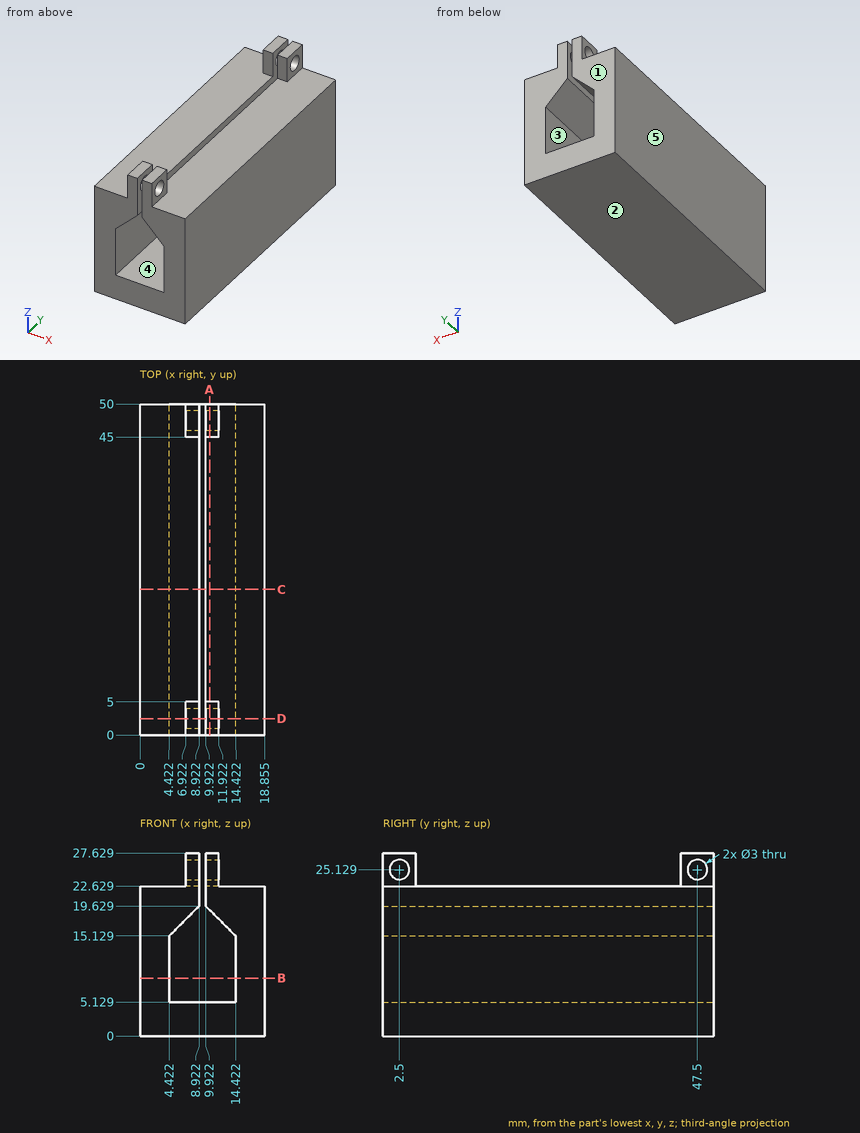
Part print with two shaded views. Sizes in mm from the minimum x, y, z corner. A direction names the side the tool comes from. Coordinates: 2 decimals unless noted, no trailing zeros. Loops run counter-clockwise (first coordinate to the right, second up) from the corner with the lowest first, then second, coordinate; pieces in that order, holes last. Notation, with made-up numbers: M -7,-13.75 L -2,-13.75 A15 cw -2,-1.75 Z; hole C 75,-27 d11. An arc over 180 degrees is marked long. Use CSV: the item, a comma, the result in double quotes. Start each with the question number.
1. Band-saw the part on C-C, the plane y = 22. List the corners of the cut face in (x, z) (1 decimal).
2. Flat gauge pins, fed straight in: pin 1 (1.5 mm diameter, centred on x = 12.5, y = 7, fed in from -Z); pin 2 (7 mm diameter, centred on x = 2.5, y = 21, fed in from +Z); pin 3 (1.5 mm diameter, centred on y = 48.5, z = 24.5, fed in from -X); pin 4 (5.5 mm diameter, centred on y = 2.5, z = 26, fed in from +X). Where does each tip first touch, or does it go through?
3. Band-saw the part on A-A, the plane x = 10.5. List the corners of the cut face in (y, z), then the cut area to 3 significant figures.
4. Band-saw the part on D-D, the plane y = 2.5. List the corners of the cut face in (x, z) (1 decimal).
5. Tool access for the marked faces 4 and 5: list every direction of +Z, -Z, +X, -X, +Y, -Y with a clear straight run to the whole face (end or side of a thin tool).
6. Two-plate mould, pull along Z, no slides. Class the marked faces 1, 2 and 3: pulls with the +Z half, pulls with the -Z half, needs draft (parallel to the pull), parting line crosses it, or undercut.
7. Probe probe 1 along X at (y, z) = (14, 6.5) (1 decimal); probe 2 along Y at (x, z) = (10, 25.75) (1 decimal); probe 3 along Z at (x, y) = (11.4, 47.5). List the from-to ranges inside material, lowest first. Write a range as [from, to].
8. Band-saw the part on B-B, the plane z = 8.75. List the corners of the cut face in (x, y) (1 decimal), then the cut area to 3 significant figures.
Entries:
1,outline,"M 0,0 L 18.9,0 L 18.9,22.6 L 9.9,22.6 L 9.9,19.6 L 14.4,15.1 L 14.4,5.1 L 4.4,5.1 L 4.4,15.1 L 8.9,19.6 L 8.9,22.6 L 0,22.6 Z"
2,pin 1,"stops at z = 0"
2,pin 2,"stops at z = 22.63"
2,pin 3,"stops at x = 6.92"
2,pin 4,"stops at x = 11.92"
3,outline,"M 0,0 L 50,0 L 50,5.13 L 0,5.13 Z; M 0,19.05 L 50,19.05 L 50,27.63 L 45,27.63 L 45,22.63 L 5,22.63 L 5,27.63 L 0,27.63 Z; hole C 2.5,25.13 d3; hole C 47.5,25.13 d3"
3,area,"471 mm2"
4,outline,"M 0,0 L 18.9,0 L 18.9,22.6 L 11.9,22.6 L 11.9,23.6 L 9.9,23.6 L 9.9,19.6 L 14.4,15.1 L 14.4,5.1 L 4.4,5.1 L 4.4,15.1 L 8.9,19.6 L 8.9,23.6 L 6.9,23.6 L 6.9,22.6 L 0,22.6 Z; M 6.9,26.6 L 8.9,26.6 L 8.9,27.6 L 6.9,27.6 Z; M 9.9,26.6 L 11.9,26.6 L 11.9,27.6 L 9.9,27.6 Z"
5,face 4,"+Y, -Y"
5,face 5,"+Z, -Z, -X, +Y, -Y"
6,face 1,"needs draft"
6,face 2,"pulls with the -Z half"
6,face 3,"undercut"
7,probe 1,"x = [0, 4.4], [14.4, 18.9]"
7,probe 2,"y = [0, 1.1], [3.9, 5], [45, 46.1], [48.9, 50]"
7,probe 3,"z = [0, 5.13], [18.15, 23.63], [26.63, 27.63]"
8,outline,"M 0,0 L 4.4,0 L 4.4,50 L 0,50 Z; M 14.4,0 L 18.9,0 L 18.9,50 L 14.4,50 Z"
8,area,"443 mm2"
